Geometry check sheet. Reference: drawing and pictorial views, mm from the part's lowest x, y, z. A direction names the side the tool comes from. Round coordinates to 2 decimals unless told otherwise and drop trailing zeros. Write each loop counter-clockwise with the first axis right and the second up, starting at its lowest first coordinate (ties: lowest second). Pieces come first, ordered by that corner, then holes.
Item 1: Material ranges on line 1 along X through (y, z) = (17, 28); line 2 along Z through (x, y) = (6.25, 38.1); line 3 along Y through (x, z) = (143, 18), recorded low to high.
Item 2: Set-up check for the marked faces 5 and 6: record each of +Z, -Z, +X, -X, +Y, -Y from which the full face is reachable in a straight line by a thin tool's end or side.
Item 3: Depth check by flat-ended pin: pin 1 (20.5 mm diameter, centred on y = 38.1, z = 38.1, fed in from -X); pin 2 (7 mm diameter, centred on x = 92, y = 70, fed in from +Z). Enter the tip coordinate at first touch or a pass-through.
Item 4: Section check B-B, the plane z = 53. Record the cut outline in (x, y), plus the area to 3 significant figures.
Item 5: Release check for a two-part mould opening along Z. For the marked faces 1, 2, 3 and 4 record: pulls with the +Z half, pulls with the -Z half, needs draft (parallel to the pull), parting line crosses it, or undercut.
Item 6: Section check D-D, the plane x = 57. Record the cut outline in (y, z).
Item 7: Section check A-A, the plane y = 62. Record the cut outline in (x, z), plus the area to 3 significant figures.
Item 8: Section check C-C, the plane y = 38.1. Record the cut outline in (x, z).
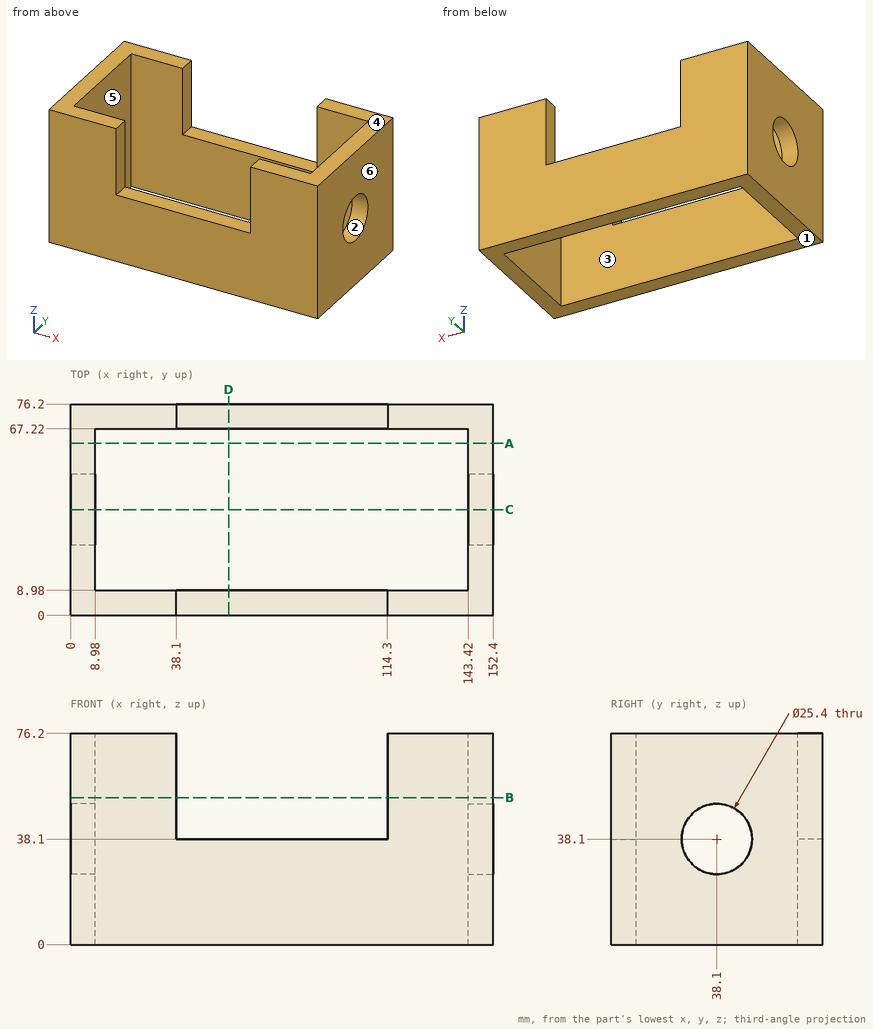
Values found:
1. line 1: x = 0 to 8.98, 143.42 to 152.4
1. line 2: z = 0 to 25.4, 50.8 to 76.2
1. line 3: y = 0 to 8.98, 67.22 to 76.2
2. face 5: +Z, -Z
2. face 6: +Z, -Z, +X, +Y, -Y
3. pin 1: passes through
3. pin 2: stops at z = 38.1
4. outline: (0, 0) - (38.1, 0) - (38.1, 8.98) - (8.98, 8.98) - (8.98, 67.22) - (38.1, 67.22) - (38.1, 76.2) - (0, 76.2) - close; (114.3, 0) - (152.4, 0) - (152.4, 76.2) - (114.3, 76.2) - (114.3, 67.22) - (143.42, 67.22) - (143.42, 8.98) - (114.3, 8.98) - close
4. area: 2,410 mm2
5. face 1: pulls with the -Z half
5. face 2: undercut
5. face 3: needs draft
5. face 4: pulls with the +Z half
6. outline: (0, 0) - (8.98, 0) - (8.98, 38.1) - (0, 38.1) - close; (67.22, 0) - (76.2, 0) - (76.2, 38.1) - (67.22, 38.1) - close
7. outline: (0, 0) - (8.98, 0) - (8.98, 76.2) - (0, 76.2) - close; (143.42, 0) - (152.4, 0) - (152.4, 76.2) - (143.42, 76.2) - close
7. area: 1,370 mm2
8. outline: (0, 0) - (8.98, 0) - (8.98, 25.4) - (0, 25.4) - close; (0, 50.8) - (8.98, 50.8) - (8.98, 76.2) - (0, 76.2) - close; (143.42, 0) - (152.4, 0) - (152.4, 25.4) - (143.42, 25.4) - close; (143.42, 50.8) - (152.4, 50.8) - (152.4, 76.2) - (143.42, 76.2) - close
